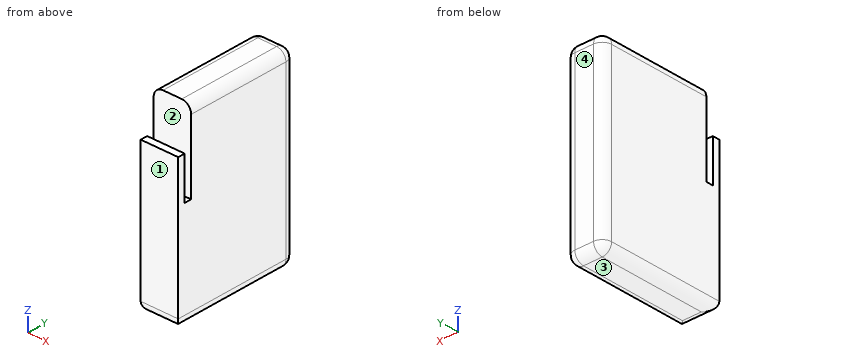
Autodesk Inventor part; units mm, degrees
ref_plane "YZ Plane" through (0, 0, 0) normal (1, 0, 0) x (0, 1, 0)
ref_plane "XZ Plane" through (0, 0, 0) normal (0, 1, 0) x (-1, 0, 0)
ref_plane "XY Plane" through (0, 0, 0) normal (0, 0, 1) x (1, 0, 0)
sketch "Sketch1" plane through (0, 0, 0) normal (1, 0, 0) x (0, 1, 0)
  line L0 (29.3798, 20) -> (5.3798, 20)
  line L1 (5.3798, 20) -> (5.3798, -20)
  line L2 (5.3798, -20) -> (29.3798, -20)
  line L3 (29.3798, -20) -> (29.3798, 20)
  line L4 (5.3798, -20) -> (2.3798, -20)
  line L5 (2.3798, -20) -> (2.3798, 2.5)
  line L6 (2.3798, 2.5) -> (5.3798, 2.5)
  line L7 (5.3798, 2.5) -> (5.3798, -20)
  line L8 (2.3798, 2.5) -> (3.8798, 2.5)
  line L9 (3.8798, 2.5) -> (3.8798, 11.5)
  line L10 (3.8798, 11.5) -> (2.3798, 11.5)
  line L11 (2.3798, 11.5) -> (2.3798, 2.5)
  point P0 (0, 0)
  point P1 (5.3798, 0)
  dimension "d0" = 24
  dimension "d1" = 40
  dimension "d2" = 3
  dimension "d3" = 22.5
  dimension "d4" = 1.5
  dimension "d5" = 9
extrude "Extrusion1" add sketch "Sketch1" along normal blind 8
fillet "Fillet1" radius 2 7 edges at (0, 17.3798, 20) (8, 17.3798, 20) (0, 15.8798, -20) (8, 15.8798, -20) (4, 2.3798, -20) (4, 29.3798, -20) (4, 29.3798, 20)
fillet "Fillet2" radius 2 6 edges at (7.4142, 28.794, 19.4142) (7.4142, 28.794, -19.4142) (8, 29.3798, 0) (0.5858, 28.794, 19.4142) (0.5858, 28.794, -19.4142) (0, 29.3798, 0)
properties part number "GATE servo motor"
CAD build for the part. Positions are in the model's coordinates, mm. Face numbers are marked on the shaded views. Round coordinates to 2 decimals unless told otherwise and drop trailing zeros. Order: outer loops, then holes, each group sorted by start corner. A loop starts at its lowest first (then second) coordinate and runs counter-clockwise, first axis right, second up.
Item 1: Mould opens along Y. For the marked faces 1, 2, 3 and 4 say: pulls with the +Y half, pulls with the -Y half, needs draft (parallel to the pull), parting line crosses it, or undercut.
Item 2: Saw through at A-A on z = 6. Write the cut outline in (x, y).
Item 3: Pin check, flat tips, straight feed: pin 1 (12 mm diameter, centred on y = 10.5, z = -9, fed in from -X); pin 2 (1.5 mm diameter, centred on x = 1, y = 8.5, fed in from +Z); pin 3 (1.2 mm diameter, centred on x = 5.5, y = 3.5, fed in from +Z). Stop position of each tip, or through.
Item 4: Saw through at C-C on x = 7. Write the cut outline in (y, z), then the cut area to 3 significant figures.
Item 5: Probe line 1 along Y through (x, z) = (2.25, 9); line 2 along X through (y, z) = (27.5, 13); line 3 along Z through (x, y) = (1, 16.5). List the from-to ranges inside material, lowest first.
Item 6: Saw through at B-B on x = 4.25. Write the cut outline in (y, z).
Reported:
1. face 1: pulls with the -Y half
1. face 2: undercut
1. face 3: needs draft
1. face 4: pulls with the +Y half
2. outline: (0, 2.38) - (8, 2.38) - (8, 3.88) - (0, 3.88) - close; (0, 5.38) - (8, 5.38) - (8, 27.38) arc R2 ccw to (6, 29.38) - (2, 29.38) arc R2 ccw to (0, 27.38) - close
3. pin 1: stops at x = 0
3. pin 2: stops at z = 19.98
3. pin 3: stops at z = 11.5
4. outline: (2.38, -18) arc R2 ccw to (3.38, -19.73) - (27.38, -19.73) arc R1.73 ccw to (29.11, -18) - (29.11, 18) arc R1.73 ccw to (27.38, 19.73) - (5.38, 19.73) - (5.38, 2.5) - (3.88, 2.5) - (3.88, 11.5) - (2.38, 11.5) - close
4. area: 1,010 mm2
5. line 1: y = 2.38 to 3.88, 5.38 to 29.38
5. line 2: x = 0 to 8
5. line 3: z = -19.73 to 19.73
6. outline: (2.38, -18) arc R2 ccw to (4.38, -20) - (27.38, -20) arc R2 ccw to (29.38, -18) - (29.38, 18) arc R2 ccw to (27.38, 20) - (5.38, 20) - (5.38, 2.5) - (3.88, 2.5) - (3.88, 11.5) - (2.38, 11.5) - close
